The model under review builds one solid part; all positions refer to its coordinate system, in mm. A direction names the side the tool comes from. Give positions to 0.01 mm unless a question says otherwise; leave off trailing zeros. Order: outer loops, then holes, each group sorted by start corner. A loop starts at its lowest first (then second) coordinate and runs counter-clockwise, first axis right, second up. Notation, with made-up numbers: (-11, 38.5) -> (31, 38.5) arc R8 ccw to (31, 46.5) -> close; hole circle Ø7 at (-2, 63.5). An arc over 180 degrees is marked (long way). Answer as a JSON object with one key per item and string values. Group by question number.
from build123d import *

# Parameters (mm, degrees)
F1_W     = 79.647951
F1_H     = 98.628715
F2_DEPTH = 25.4
F3_DEPTH = 25.4


with BuildPart() as f2:
    # F1 (on Top) → F2 (new body)
    with BuildSketch(Plane.XY):
        with Locations((3.260706, 1.626015)):
            Rectangle(F1_W, F1_H)
    extrude(amount=F2_DEPTH)

    # F0 (on Front) → F3 (join)
    with BuildSketch(Plane.XZ):
        with BuildLine():
            Line((21.648072, -16.353669), (31.325075, 3.271477))
            ThreePointArc((31.325075, 3.271477), (7.739275, 0.538226), (0.530634, -22.084684))
            Line((0.530634, -22.084684), (21.648072, -16.353669))
        make_face()
        Polygon((43.848254, 28.668722), (-38.244482, 28.668722), (-38.244482, -32.607779), align=None)
        with BuildLine():
            Line((31.325075, 3.271477), (43.848254, 28.668722))
            Line((43.848254, 28.668722), (-38.244482, -32.607779))
            Line((-38.244482, -32.607779), (0.530634, -22.084684))
            ThreePointArc((0.530634, -22.084684), (7.739275, 0.538226), (31.325075, 3.271477))
        make_face()
        with BuildLine():
            ThreePointArc((43.529359, -16.353669), (40.22946, -4.798465), (31.325075, 3.271477))
            Line((31.325075, 3.271477), (21.648072, -16.353669))
            Line((21.648072, -16.353669), (0.530634, -22.084684))
            ThreePointArc((0.530634, -22.084684), (24.53892, -38.043153), (43.529359, -16.353669))
        make_face()
    extrude(amount=F3_DEPTH)


solid = f2.part
1. Draft analysis for pull direction X (two halves, no side actions). For faces 1 (the flat face through (3, -47.688, 13)), 2 (the flat face through (-36.563, 25, 13)), 3 (the flat face through (-19.13, -12.52, -27.42)), state which applies: pulls with the +X half, pulls with the -X half, needs draft (parallel to the pull), parting line crosses it, or undercut.
2. Take a section at B-B on x = -14. Give the boundary of the cut face in (y, z), plus the area to 3 significant figures.
3. For probe 1 along Y at (x, z) = (36, -0.5); probe 2 along Z at (x, y) = (32.5, -33.5); probe 3 along X at (y, z) = (-14, 2), list the stretches that pass through material, from the lowest coordinate up. Write a range as [from, to].
4. For pin 1 (1 mm diameter, centred on x = 14, y = 22.5, fed in from +Z); pin 2 (6 mm diameter, centred on x = 7.5, z = -20.5, fed in from -Y); pin 3 (6.5 mm diameter, centred on y = -34, z = 15, fed in from -X), all flat-tipped, find the tip position at first contact; note any pin that passes through.
5. Machinability: for faces 4 (the flat face through (43.085, 1, 13)), 5 (the flat face through (3, 50.94, 13)), 6 (the flat face through (-36.563, -37, 13)), which of the approach directions +Z, -Z, +X, -X, +Y, -Y give a long, thin tool a straight path to every point of the face, cutting with its end or side? Answer none if there is none.
6. Take a section at A-A on y = -17. Give the boundary of the cut face in (x, z), plus the area to 3 significant figures.
7. Take a section at C-C on z = 12.5. Give the boundary of the cut face in (x, y).
8. Take a section at D-D on x = -22.5. Give the boundary of the cut face in (y, z).
Checks:
{
 "1": {"face 1": "needs draft", "face 2": "pulls with the -X half", "face 3": "undercut"},
 "2": {"outline": "(-47.69, 0) -> (-25.4, 0) -> (-25.4, -26.03) -> (0, -26.03) -> (0, 0) -> (50.94, 0) -> (50.94, 25.4) -> (0, 25.4) -> (0, 28.67) -> (-25.4, 28.67) -> (-25.4, 25.4) -> (-47.69, 25.4) -> close", "area": "3,250 mm2"},
 "3": {"probe 1": "y = [-25.4, 0]", "probe 2": "z = [0, 25.4]", "probe 3": "x = [-38.24, 43.08]"},
 "4": {"pin 1": "stops at z = 25.4", "pin 2": "stops at y = -25.4", "pin 3": "stops at x = -36.56"},
 "5": {"face 4": "+X, +Y, -Y", "face 5": "+Z, -Z, +X, -X, +Y", "face 6": "+Z, -Z, -X, -Y"},
 "6": {"outline": "(-38.24, -32.61) -> (0.53, -22.08) arc R21.88 ccw to (43.53, -16.35) arc R21.88 ccw to (36.19, 0) -> (43.08, 0) -> (43.08, 25.4) -> (42.24, 25.4) -> (43.85, 28.67) -> (-38.24, 28.67) -> close", "area": "4,810 mm2"},
 "7": {"outline": "(-38.24, -25.4) -> (-36.56, -25.4) -> (-36.56, -47.69) -> (43.08, -47.69) -> (43.08, 50.94) -> (-36.56, 50.94) -> (-36.56, 0) -> (-38.24, 0) -> close"},
 "8": {"outline": "(-47.69, 0) -> (-25.4, 0) -> (-25.4, -28.33) -> (0, -28.33) -> (0, 0) -> (50.94, 0) -> (50.94, 25.4) -> (0, 25.4) -> (0, 28.67) -> (-25.4, 28.67) -> (-25.4, 25.4) -> (-47.69, 25.4) -> close"}
}
